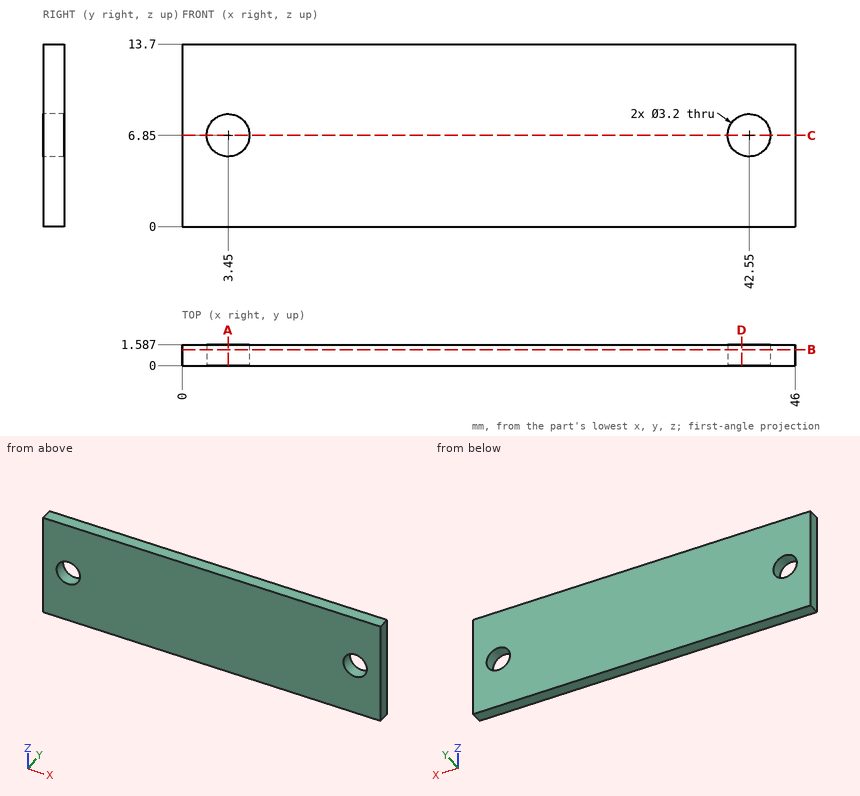
Source: three-view drawing plus pictorial views. Frame: mm from the lowest corner of the part. Give positions to 0.01 mm unless a question says otherwise; leave off trailing zeros. Loops run counter-clockwise (first coordinate to the right, second up) from the corner with the lowest first, then second, coordinate; pieces in that order, holes last. Notation, with made-up numbers: M -23.75,39 L -13.75,39 A20 cw -13.75,71 Z; hole C -13,81.25 d5. An arc over 180 degrees is marked long. Put each result on its own line as item: value.
Q1. Section A-A (x = 3.45). Return the cut outline in (y, z).
Response values:
outline: M 0,0 L 1.59,0 L 1.59,5.25 L 0,5.25 Z; M 0,8.45 L 1.59,8.45 L 1.59,13.7 L 0,13.7 Z
Q2. Pin query (flat end, axial travel): P1, Ø3, axis at x = 42.55, z = 6.85, coming from the -Y side. Return the tip coordinate at first contact, or that it passes through.
Response values:
P1: passes through
Q3. Line query: probe 1 along Z at (x, y) = (42.55, 1.3); probe 2 along Z at (x, y) = (2.5, 0.2) (1 decimal). Output: solid intervals per line, ascending. Write a range as [from, to].
Response values:
probe 1: z = [0, 5.25], [8.45, 13.7]
probe 2: z = [0, 5.6], [8.1, 13.7]
Q4. Section C-C (z = 6.85). Return the cut outline in (x, y).
Response values:
outline: M 0,0 L 1.85,0 L 1.85,1.59 L 0,1.59 Z; M 5.05,0 L 40.95,0 L 40.95,1.59 L 5.05,1.59 Z; M 44.15,0 L 46,0 L 46,1.59 L 44.15,1.59 Z
Q5. Section D-D (x = 42). Return the cut outline in (y, z).
Response values:
outline: M 0,0 L 1.59,0 L 1.59,5.35 L 0,5.35 Z; M 0,8.35 L 1.59,8.35 L 1.59,13.7 L 0,13.7 Z
Q6. Section B-B (y = 1.2). Return the cut outline in (x, z), and give its area (3 significant figures).
Response values:
outline: M 0,0 L 46,0 L 46,13.7 L 0,13.7 Z; hole C 3.45,6.85 d3.2; hole C 42.55,6.85 d3.2
area: 614 mm²
